Could you check a few things on this drawing? It's one solid part, dimensions in mm from its lowest x, y, z. Coordinates: 2 decimals unless noted, no trailing zeros. Order: outer loops, then holes, each group sorted by start corner. A loop starts at its lowest first (then second) coordinate and runs counter-clockwise, first axis right, second up. Notation, with made-up numbers: M -31,74 L 2,74 A13 cw 2,81 Z; hole C 50.5,-31 d5. An arc over 180 degrees is marked long. One line per question, with ' | ' between items. Start each with the question number.
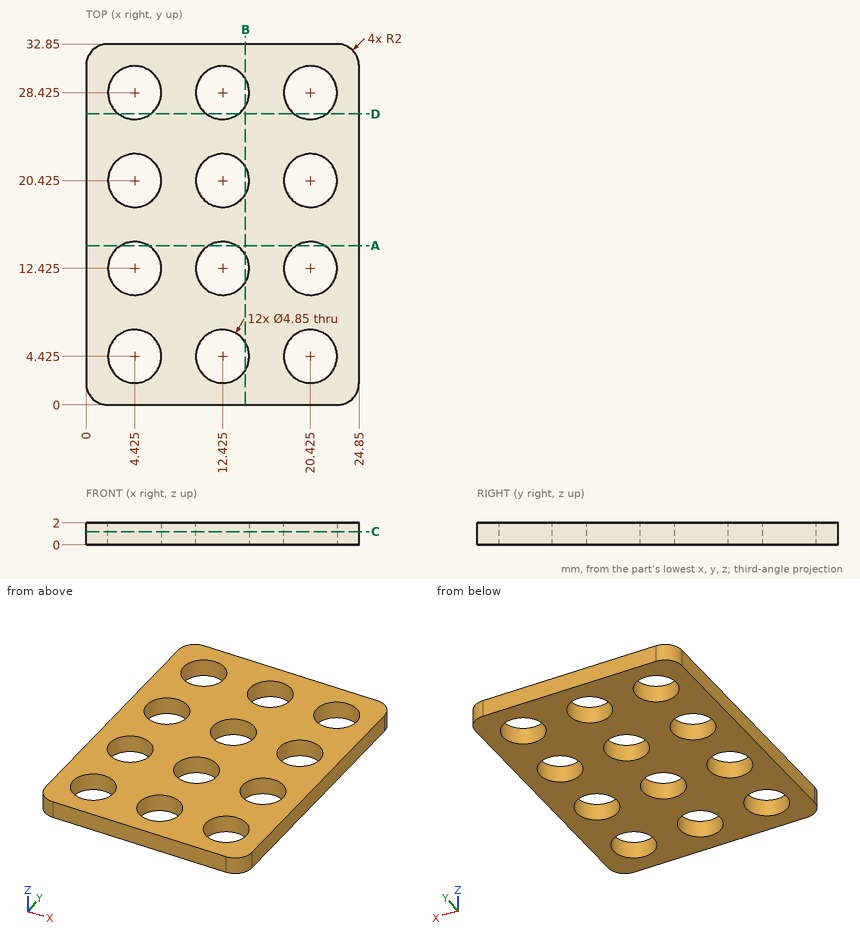
1. Imagine slicing it at B-B (x = 14.5). List the corners of the cut face in (y, z) for me.
2. I need wall thicknesses on line 1 (Y direction, x = 12.5, z = 0.4); line 2 (X direction, y = 4.5, z = 0.5); line 3 (Y direction, x = 10.5, z = 0.1). Which ranges of each line are inside material? Lowest first, please.
3. Imagine slicing it at D-D (y = 26.5). List the corners of the cut face in (x, z) for me, then the cut area to 3 significant figures.
4. Imagine slicing it at A-A (y = 14.5). List the corners of the cut face in (x, z) for me, then the cut area to 3 significant figures.
5. Imagine slicing it at C-C (z = 1.2). Count the separate pieces of the cut face and the enclosed holes in it, then the cut area to 3 significant figures.
6. Will this pin go through, and if not, where does the flat tip stop? pin 1 (4.5 mm diameter, centred on x = 4.425, y = 20.425, fed in from -Z).
Entries:
1) outline: M 0,0 L 3.17,0 L 3.17,2 L 0,2 Z; M 5.68,0 L 11.17,0 L 11.17,2 L 5.68,2 Z; M 13.68,0 L 19.17,0 L 19.17,2 L 13.68,2 Z; M 21.68,0 L 27.17,0 L 27.17,2 L 21.68,2 Z; M 29.68,0 L 32.85,0 L 32.85,2 L 29.68,2 Z
2) line 1: 0 to 2, 6.85 to 10, 14.85 to 18, 22.85 to 26, 30.85 to 32.85 | line 2: 0 to 2, 6.85 to 10, 14.85 to 18, 22.85 to 24.85 | line 3: 0 to 2.95, 5.9 to 10.95, 13.9 to 18.95, 21.9 to 26.95, 29.9 to 32.85
3) outline: M 0,0 L 2.95,0 L 2.95,2 L 0,2 Z; M 5.9,0 L 10.95,0 L 10.95,2 L 5.9,2 Z; M 13.9,0 L 18.95,0 L 18.95,2 L 13.9,2 Z; M 21.9,0 L 24.85,0 L 24.85,2 L 21.9,2 Z | area: 32.0 mm²
4) outline: M 0,0 L 3.17,0 L 3.17,2 L 0,2 Z; M 5.68,0 L 11.17,0 L 11.17,2 L 5.68,2 Z; M 13.68,0 L 19.17,0 L 19.17,2 L 13.68,2 Z; M 21.68,0 L 24.85,0 L 24.85,2 L 21.68,2 Z | area: 34.6 mm²
5) separate pieces: 1 | enclosed holes: 12 | area: 591 mm²
6) pin 1: through
